For this review, take the finished solid that the model builds, in its own axes (mm). A direction names the side the tool comes from. Coordinates: 2 decimals unless noted, no trailing zeros. Write each loop counter-clockwise with the first axis right and the second up, starting at its lowest first coordinate (ties: lowest second). Pieces come first, ordered by that corner, then holes. Notation, with made-up numbers: (-33, -8.5) - (-24, -8.5) arc R15 ccw to (-24, -4.5) - close; hole circle Ø5 at (46, 68.5). An arc over 180 degrees is marked (long way). Use one line per item in the form item = value. Start each with the question number.
1) Mouldability with a two-part tool opening along Y and no side actions: class faces 4 (the flat face through (8, 25.4, 17)), 5 (the cylindrical face through (126.34, 112.75, 11.46)), 6 (the flat face through (127, 63, 16)) as pulls with the +Y half, pulls with the -Y half, needs draft (parallel to the pull), parting line crosses it, or undercut.
2) We need section D-D (y = 37). Give the boundary of the cut face in (x, z) (3 decimals).
3) Insertion check: P1, Ø2.5, axis at y = 114.3, z = 11.11, coming from the +X side; P2, Ø2, axis at x = 72, y = 96.5, coming from the +Z side (3 decimals). Each pin has a flat end and moves straight along its axis. Give the tip position at first contact, or say it passes through.
4) For L1, parallel to Z at x = 126.45, y = 114.3 (3 decimals); L2, parallel to X at y = 31.75, z = 24.5; L3, parallel to Y at x = 117, z = 26.5 (3 decimals), list the stretches that pass through material, from the lowest coordinate up. Write a range as from..to.
5) Tool access review of faces 1 (the conical face through (125.537, 14.347, 11.478)), 2 (the flat face through (3.175, 14, 17)), 3 (the cylindrical face through (0.66, 12.22, 9.6)): name each direction out of +Z, -Z, +X, -X, +Y, -Y from which nothing blocks a thin tool from reaching the whole face with its end or side.
6) We need section A-A (z = 29). Count the separate pieces of the cut face and the enclosed holes in it, plus the area to 3 significant figures.
7) We need section C-C (x = 48). Give the boundary of the cut face in (y, z) (3 decimals).
Autodesk Inventor part; units mm, degrees
ref_plane "Work Plane1" through (63.5, 0, 0) normal (1, 0, 0) x (0, 0, -1)
ref_plane "YZ Plane" through (0, 0, 0) normal (1, 0, 0) x (0, 1, 0)
ref_plane "XZ Plane" through (0, 0, 0) normal (0, 1, 0) x (-1, 0, 0)
sketch "Sketch1" plane through (0, 0, 0) normal (0, 0, 1) x (1, 0, 0)
  line L0 (0, 0) -> (127, 0)
  line L1 (127, 0) -> (127, 127)
  line L2 (127, 127) -> (0, 127)
  line L3 (0, 127) -> (0, 0)
  dimension "d0" = 127
  dimension "d1" = 127
extrude "Extrusion1" add sketch "Sketch1" along normal blind 31.75
shell "Shell1" thickness 3.175 removed faces 1 at (42.3333, 84.6667, 31.75)
sketch "Sketch3" plane through (3.175, 3.175, 3.175) normal (1, 0, 0) x (0, 0, -1)
  line L0 (0, 0) -> (-28.575, 0) construction
  line L1 (-14.2875, 0) -> (-14.2875, 120.65) construction
  line L2 (0, 120.65) -> (-28.575, 120.65) construction
  line L3 (-14.2875, 120.65) -> (-20.6375, 120.65) construction
  line L4 (-20.6375, 120.65) -> (-20.6375, 111.125) construction
  line L5 (-20.6375, 111.125) -> (-14.2875, 111.125) construction
  line L6 (-14.2875, 111.125) -> (-14.2875, 120.65) construction
  line L7 (-14.2875, 120.65) -> (-7.9375, 120.65) construction
  line L8 (-7.9375, 120.65) -> (-7.9375, 111.125) construction
  line L9 (-7.9375, 111.125) -> (-14.2875, 111.125) construction
  line L10 (-14.2875, 111.125) -> (-14.2875, 120.65) construction
  line L11 (-14.2875, 0) -> (-20.6375, 0) construction
  line L12 (-20.6375, 0) -> (-20.6375, 9.525) construction
  line L13 (-20.6375, 9.525) -> (-14.2875, 9.525) construction
  line L14 (-14.2875, 9.525) -> (-14.2875, 0) construction
  line L15 (-14.2875, 0) -> (-7.9375, 0) construction
  line L16 (-7.9375, 0) -> (-7.9375, 9.525) construction
  line L17 (-7.9375, 9.525) -> (-14.2875, 9.525) construction
  line L18 (-14.2875, 9.525) -> (-14.2875, 0) construction
  point P0 (3.175, -3.175)
  dimension "d5" = 6.35
  dimension "d6" = 9.525
  dimension "d7" = 6.35
  dimension "d8" = 6.35
  dimension "d9" = 9.525
  dimension "d10" = 6.35
  dimension "d11" = 9.525
hole "Hole1" at (3.175, 12.7, 23.8125) at (3.175, 12.7, 11.1125) at (3.175, 114.3, 23.8125) at (3.175, 114.3, 11.1125) direction (-1, 0, 0) diameter 3.175 depth 15.6718 tip angle 118 countersink diameter 6.35 countersink angle 82
ref_plane "Work Plane1" through (63.5, 0, 0) normal (1, 0, 0) x (0, 0, -1)
sketch "Sketch4" plane through (3.175, 3.175, 3.175) normal (0, 0, 1) x (1, 0, 0)
  line L0 (0, 0) -> (0, 120.65) construction
  line L1 (0, 120.65) -> (0, 98.425) construction
  line L2 (0, 0) -> (120.65, 0) construction
  line L3 (0, 0) -> (0, 22.225) construction
  line L4 (0, 98.425) -> (9.525, 98.425)
  line L5 (9.525, 98.425) -> (9.525, 22.225)
  line L6 (9.525, 22.225) -> (0, 22.225)
  line L7 (0, 22.225) -> (0, 98.425)
  point P0 (-3.175, -3.175)
  dimension "d19" = 22.225
  dimension "d20" = 22.225
  dimension "d21" = 9.525
extrude "Extrusion2" add sketch "Sketch4" along normal up to surface (28.575 mm away)
sketch "Sketch5" plane through (0, 0, 31.75) normal (0, 0, 1) x (1, 0, 0)
  line L0 (12.7, 101.6) -> (12.7, 25.4) construction
  line L1 (12.7, 25.4) -> (6.35, 25.4) construction
  line L2 (6.35, 25.4) -> (6.35, 31.75) construction
  line L3 (6.35, 31.75) -> (12.7, 31.75) construction
  line L4 (12.7, 31.75) -> (12.7, 25.4) construction
  line L5 (12.7, 101.6) -> (6.35, 101.6) construction
  line L6 (6.35, 101.6) -> (6.35, 95.25) construction
  line L7 (6.35, 95.25) -> (12.7, 95.25) construction
  line L8 (12.7, 95.25) -> (12.7, 101.6) construction
  point P0 (0, 0)
  dimension "d24" = 6.35
  dimension "d25" = 6.35
  dimension "d26" = 6.35
  dimension "d27" = 6.35
hole "Hole2" at (6.35, 95.25, 31.75) at (6.35, 31.75, 31.75) direction (0, 0, -1) diameter 3.175 depth 12.7 tip angle 118
mirror "Mirror2" about plane through (63.5, 0, 0) normal (1, 0, 0) of "Hole1", "Extrusion2", "Hole2"
fillet "Fillet1" radius 3.175 12 edges at (3.175, 123.825, 17.4625) (12.7, 101.6, 17.4625) (3.175, 101.6, 17.4625) (12.7, 25.4, 17.4625) (3.175, 25.4, 17.4625) (3.175, 3.175, 17.4625) (123.825, 3.175, 17.4625) (123.825, 25.4, 17.4625) (114.3, 25.4, 17.4625) (114.3, 101.6, 17.4625) (123.825, 101.6, 17.4625) (123.825, 123.825, 17.4625)
properties part number "wheel core"
Determined:
q1.face_4 = undercut
q1.face_5 = undercut
q1.face_6 = needs draft
q2.outline = (0, 0) - (127, 0) - (127, 31.75) - (114.3, 31.75) - (114.3, 3.175) - (12.7, 3.175) - (12.7, 31.75) - (0, 31.75) - close
q3.P1 = through
q3.P2 = 3.175
q4.L1 = 0..9.525, 12.7..22.225, 25.4..31.75
q4.L2 = 0..4.76, 7.94..12.7, 114.3..119.06, 122.24..127
q4.L3 = 0..3.175, 25.436..101.564, 123.825..127
q5.face_1 = none
q5.face_2 = +Z
q5.face_3 = +X, -X
q6.separate_pieces = 1
q6.enclosed_holes = 5
q6.area = 3,000 mm²
q7.outline = (0, 0) - (127, 0) - (127, 31.75) - (123.825, 31.75) - (123.825, 3.175) - (3.175, 3.175) - (3.175, 31.75) - (0, 31.75) - close
